Design review of the part built by this model. Coordinates are the model's own, in mm. Coordinates: 2 decimals unless noted, no trailing zeros. Order: outer loops, then holes, each group sorted by start corner. A loop starts at its lowest first (then second) coordinate and runs counter-clockwise, first axis right, second up. Notation, with made-up numbers: (14.5, 31.25) - (63.5, 31.25) arc R26 cw to (63.5, 57.25) - close; hole circle Ø3 at (12, 59.5). An arc over 180 degrees is marked (long way). Write item = value, one per line. Start each with the question number.
```python
from build123d import *

# Parameters (mm, degrees)
BOSS_EXTRUDE1_DEPTH      = 304.8
BOSS_EXTRUDE1_DEPTH_BACK = 304.8
SKETCH4_R                = 4.7625
CHAMFER1_SIZE            = 0.24765
CUT_EXTRUDE1_START       = 4
CUT_EXTRUDE1_DEPTH       = 1


with BuildPart() as part:
    # Sketch4 → Boss-Extrude1 (new, two sides: drawn at the far end of the back side and taken through both)
    with BuildSketch(Plane(origin=(0, 0, 0), x_dir=(0, 0, -1), z_dir=(1, 0, 0)).offset(-BOSS_EXTRUDE1_DEPTH_BACK)):
        with Locations(Location((0, 0, 0), (0, 0, 180))):
            Circle(SKETCH4_R)
    extrude(amount=BOSS_EXTRUDE1_DEPTH + BOSS_EXTRUDE1_DEPTH_BACK)

    # Chamfer1
    chamfer1_edges = [part.edges().sort_by_distance(p)[0] for p in [
        (-304.8, 0, -4.7625),
        (304.8, 0, -4.7625),
    ]]
    chamfer(chamfer1_edges, length=CHAMFER1_SIZE)

    # Sketch5 → Cut-Revolve1 (revolve, cut)
    with BuildSketch(Plane.XY, mode=Mode.PRIVATE) as cut_revolve1_sk:
        Polygon((304.8, 0), (120.65, 0), (120.65, 3.238), (119.888, 4), (95.25, 4), (95.25, 4.3815), (94.869, 4.7625), (304.8, 4.7625), align=None)
    revolve(cut_revolve1_sk.sketch.rotate(Axis((120.65, 0, 0), (1, 0, 0)), 90), axis=Axis((120.65, 0, 0), (1, 0, 0)), mode=Mode.SUBTRACT)

    # Sketch6 → Cut-Extrude1 (cut)
    with BuildSketch(Plane(origin=(0, 0, 0), x_dir=(1, 0, 0), z_dir=(0, 1, 0)).offset(CUT_EXTRUDE1_START)):
        with BuildLine():
            Line((120.65, -1), (98.425, -1))
            ThreePointArc((98.425, -1), (97.425, 0), (98.425, 1))
            Line((98.425, 1), (120.65, 1))
            ThreePointArc((120.65, 1), (121.65, 0), (120.65, -1))
        make_face()
    extrude(amount=-CUT_EXTRUDE1_DEPTH, mode=Mode.SUBTRACT)


solid = part.part
```
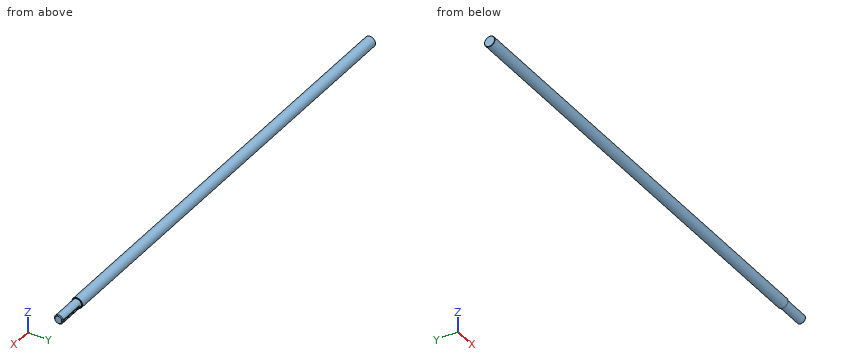
Item 1: Add section A-A on x = -91. Give the boundary of the cut face in (y, z) (1 decimal).
Item 2: For line 1 (Z direction, x = -77, y = -2); line 2 (Y direction, x = -207, z = -3.5); line 3 (Y direction, x = -196, z = 2.5), list the stretches that pass through material, from the lowest coordinate up.
Item 3: For P1, Ø1, axis at x = 108, y = 3.5, coming from the +Z side; P2, Ø0.6, axis at x = 113.5, z = 0, coming from the +Y side; P3, Ø1, axis at y = 3.5, z = 3, coming from the +X side, all flat-tipped, find the tip position at first contact; note any pin that passes through.
Worked out:
q1.outline = circle Ø9.5 at (0, 0)
q2.line_1 = -4.32 to 4.32
q2.line_2 = -3.23 to 3.23
q2.line_3 = -4.05 to 4.05
q3.P1 = 2.65
q3.P2 = 3
q3.P3 = 95.25
